Can you work these out from the model? Positions are in its coordinate system, mm. Face numbers are marked on the shaded views. A direction names the side the tool comes from. Round coordinates to 2 decimals unless told otherwise and drop trailing zeros. Loops run counter-clockwise (first coordinate to the right, second up) from the corner with the lowest first, then second, coordinate; pieces in that order, holes last. Notation, with made-up numbers: M 44.25,19.5 L 52.25,19.5 A31 cw 52.25,44.5 Z; hole C 51,-33 d11. An arc over 180 degrees is marked long. Return JSON: item names as keys, results as strings.
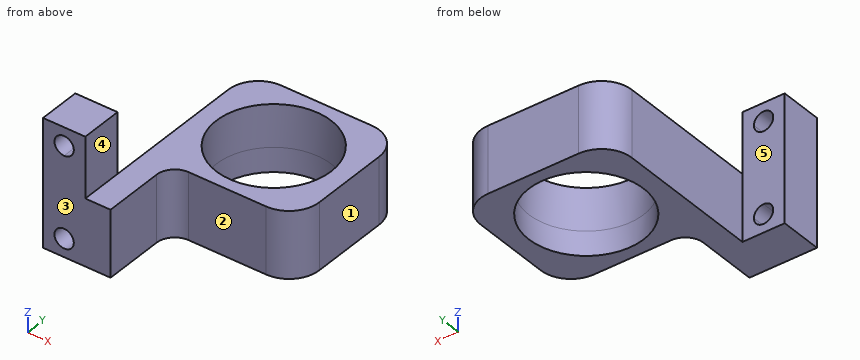
```python
from build123d import *

# Parameters (mm, degrees)
F0_W     = 32
F0_H     = 36
F1_DEPTH = 4
F2_R     = 9.5
F2_W     = 7
F2_H     = 29
F2_W_2   = 20.817460835
F2_H_2   = 13
F3_DEPTH = 25
F4_W     = 7
F4_H     = 7
F4_R     = 9.5
F5_DEPTH = 7
F6_DEPTH = 17
F8_DEPTH = 25
F9_R     = 5
F10_R    = 3


# Not quite as in the source:
# - a feature of the source that left no trace in its solid (it failed there, or was rolled back) is left out


with BuildPart() as f1:
    # F0 (on Top) → F1 (new body)
    with BuildSketch(Plane.XY):
        with Locations((16, 18)):
            Rectangle(F0_W, F0_H)
    extrude(amount=F1_DEPTH)

    # F2 (on face) → F3 (cut)
    with BuildSketch(Plane.XY.offset(4)):
        with Locations((19.5, 24.5)):
            Circle(F2_R)
        with Locations((3.5, 21.5)):
            Rectangle(F2_W, F2_H)
        with Locations((21.5912695825, 6.5)):
            Rectangle(F2_W_2, F2_H_2)
    extrude(amount=-F3_DEPTH, mode=Mode.SUBTRACT)

    # F4 (on face) → F5 (join)
    with BuildSketch(Plane.XY.offset(4)):
        with Locations((3.5, 3.5)):
            Rectangle(F4_W, F4_H)
        Polygon((7, 36), (7, 7), (7, 0), (11.182539165, 0), (11.182539165, 13), (32, 13), (32, 36), align=None)
        with Locations((19.5, 24.5)):
            Circle(F4_R, mode=Mode.SUBTRACT)
    extrude(amount=F5_DEPTH)

    # F4 (on face) → F6 (join)
    with BuildSketch(Plane.XY.offset(4)):
        with Locations((3.5, 3.5)):
            Rectangle(F4_W, F4_H)
    extrude(amount=F6_DEPTH)

    # F7 (on face) → F8 (cut)
    with BuildSketch(Plane.XZ):
        with BuildLine():
            ThreePointArc((5.1, 3), (4.6313708499, 4.1313708499), (3.5, 4.6))
            ThreePointArc((3.5, 4.6), (2.3686291501, 1.8686291501), (5.1, 3))
        make_face()
        with BuildLine():
            ThreePointArc((5.1, 18), (2.3686291501, 19.1313708499), (3.5, 16.4))
            ThreePointArc((3.5, 16.4), (4.6313708499, 16.8686291501), (5.1, 18))
        make_face()
    extrude(amount=-F8_DEPTH, mode=Mode.SUBTRACT)

    # F9
    f9_edges = [f1.edges().sort_by_distance(p)[0] for p in [
        (32, 36, 5.5),
        (7, 36, 5.5),
        (32, 13, 5.5),
    ]]
    fillet(f9_edges, radius=F9_R)

    # F10
    f10_edges = [f1.edges().sort_by_distance(p)[0] for p in [
        (11.182539, 13, 5.5),
    ]]
    fillet(f10_edges, radius=F10_R)


solid = f1.part
```
Q1. Suppose I cut it at D-D, the plane y = 8. Please give me the cut outline in (x, z).
Results:
{"outline": "M 7,0 L 11.18,0 L 11.18,11 L 7,11 Z"}
Q2. If I drill on line 1 along Z through (x, y) = (3.5, 5); line 2 along Y through (x, z) = (19.5, 1.15); line 3 along Y through (x, z) = (4.5, 13.5), over which ranges is the centre line in solid material (lowest first)?
Results:
{"line 1": "z = 0 to 1.4, 4.6 to 16.4, 19.6 to 21", "line 2": "y = 13 to 15, 34 to 36", "line 3": "y = 0 to 7"}
Q3. Suppose I cut it at C-C, the plane y = 24.5. Please give me the cut outline in (x, z), plus the area to 3 significant figures.
Results:
{"outline": "M 7,0 L 10,0 L 10,11 L 7,11 Z; M 29,0 L 32,0 L 32,11 L 29,11 Z", "area": "66.0 mm2"}
Q4. I'm going to push flat-ended pins straight in: pin 1 Ø5 at (y, z) = (7, 10) entering from +X; pin 2 Ø5.5 at (x, z) = (18.5, 5.5) entering from -Y; pin 3 Ø12.5 at (x, y) = (13.5, 17.5) entering from +Z. Where does each tip first touch, or does it pass through?
Results:
{"pin 1": "stops at x = 11.18", "pin 2": "stops at y = 13", "pin 3": "stops at z = 11"}
Q5. Suppose I cut it at A-A, the plane z = 8.75. Please give me the cut outline in (x, y).
Results:
{"outline": "M 0,0 L 11.18,0 L 11.18,10 A3 cw 14.18,13 L 27,13 A5 ccw 32,18 L 32,31 A5 ccw 27,36 L 12,36 A5 ccw 7,31 L 7,7 L 0,7 Z; hole C 19.5,24.5 d19"}
Q6. Suppose I cut it at B-B, the plane x = 19.5. Please give me the cut outline in (y, z).
Results:
{"outline": "M 13,0 L 15,0 L 15,11 L 13,11 Z; M 34,0 L 36,0 L 36,11 L 34,11 Z"}
Q7. On a 3-axis mill with a long thin cutter (end or side, diameter ignored), from which of +Z, -Z, +X, -X, +Y, -Y can I reach the whole of each face in a straight line? I mean the marked faces 1, 2, 3, 4 and 5. Say none if no direction works.
Results:
{"face 1": "+Z, -Z, +X, +Y, -Y", "face 2": "+Z, -Z, +X, -Y", "face 3": "+Z, -Z, +X, -X, -Y", "face 4": "+Z, +X, +Y, -Y", "face 5": "+Z, -Z, -X, +Y"}
